```python
from build123d import *

# Parameters (mm, degrees)
SKETCH1_R                 = 3.96875
SKETCH1_R_2               = 1.5875
BODY_DEPTH                = 38.1
SKETCH1_3_R               = 1.5875
POT_SHAFT_OPENING_DEPTH   = 15.24
F_6_32_TAPPED_HOLE1_D     = 2.7051
F_6_32_TAPPED_HOLE1_DEPTH = 3.81
F_6_32_TAPPED_HOLE1_TIP   = 0.81269403


with BuildPart() as part:
    # Sketch1 → Body (new body)
    # profile 1 of 2: a face of its own
    with BuildSketch(Plane.XY):
        Circle(SKETCH1_R)
        Circle(SKETCH1_R_2, mode=Mode.SUBTRACT)
    # profile 2 of 2: a face of its own
    with BuildSketch(Plane.XY):
        Circle(SKETCH1_R_2)
    extrude(amount=-BODY_DEPTH)

    # Sketch1_3 → POT Shaft Opening (cut)
    with BuildSketch(Plane.XY):
        Circle(SKETCH1_3_R)
    extrude(amount=-POT_SHAFT_OPENING_DEPTH, mode=Mode.SUBTRACT)

    # 6-32 Tapped Hole1
    with Locations(Plane(origin=(3.96875, 0, 0), x_dir=(0, 0, -1), z_dir=(1, 0, 0))):
        with Locations((4.7625, 0)):
            Hole(F_6_32_TAPPED_HOLE1_D / 2, depth=F_6_32_TAPPED_HOLE1_DEPTH)
            with Locations((0, 0, -(F_6_32_TAPPED_HOLE1_DEPTH + F_6_32_TAPPED_HOLE1_TIP / 2))):  # 118° drill point
                Cone(0, F_6_32_TAPPED_HOLE1_D / 2, F_6_32_TAPPED_HOLE1_TIP, mode=Mode.SUBTRACT)


solid = part.part
```
Input: part model. Units: mm. Frame: model coordinates. A direction names the side the tool comes from. Round coordinates to 2 decimals unless told otherwise and drop trailing zeros. Order: outer loops, then holes, each group sorted by start corner. A loop starts at its lowest first (then second) coordinate and runs counter-clockwise, first axis right, second up. Notation, with made-up numbers: (-25.75, 16.25) - (19.25, 16.25) arc R15 ccw to (19.25, 32.25) - close; hole circle Ø9 at (42, 6). An arc over 180 degrees is marked (long way). One line per question, with ' | ' between items. Start each with the question number.
1) Contact query for flat-ended pins moving along their axis: P1, Ø1.5, axis at x = 2, z = -13, coming from the +Y side; P2, Ø2, axis at x = -2.5, z = -21, coming from the +Y side. Output: stop coordinate, or through.
2) Set-up query: faces 1 (the flat face through (0, 0, -15.24)), 2 (the flat face through (2, 0, 0)). Return all of +Z, -Z, +X, -X, +Y, -Y with unobstructed straight access to the full face (end or side cutting, diameter ignored); none if empty.
3) Cut plane D-D, the plane x = 2.5. Return the cut outline in (y, z).
4) Pull-direction query (X, two-part tool) for faces 3 (the cylindrical face through (-0.86, -3.874, -18.783)), 4 (the cylindrical face through (-1.586, 0.07, -7.513)), 5 (the cylindrical face through (2.38, 1.34, -4.94)); classes: +X half, -X half, draft (parallel to the pull), parting line (faces both ways), or undercut.
5) Cut plane A-A, the plane y = 0. Return the cut outline in (x, z), then the cut area to 3 significant figures.
6) Cut plane C-C, the plane z = -6.5. Return the cut outline in (x, y) (1 decimal).
7) Cut plane B-B, the plane x = 0. Return the cut outline in (y, z).
8) Ray query, probe 1 along Z at (x, y) = (2.75, 0); probe 2 along Y at (x, z) = (0, -5.75); probe 3 along X at (y, z) = (-0.75, -10). Return the intervals inside material, ascending.
Worked out:
1) P1: stops at y = 3.77 | P2: stops at y = 3.67
2) face 1: +Z | face 2: +Z, +X, -X, +Y, -Y
3) outline: (-3.08, -38.1) - (3.08, -38.1) - (3.08, 0) - (-3.08, 0) - close; hole circle Ø2.71 at (0, -4.76)
4) face 3: parting line | face 4: undercut | face 5: draft
5) outline: (-3.97, -38.1) - (3.97, -38.1) - (3.97, -6.12) - (1.59, -6.12) - (1.59, -15.24) - (-1.59, -15.24) - (-1.59, 0) - (-3.97, 0) - close; (1.59, -3.41) - (3.97, -3.41) - (3.97, 0) - (1.59, 0) - close | area: 248 mm^2
6) outline: circle Ø7.9 at (0, 0); hole circle Ø3.2 at (0, 0)
7) outline: (-3.97, -38.1) - (3.97, -38.1) - (3.97, 0) - (1.59, 0) - (1.59, -15.24) - (-1.59, -15.24) - (-1.59, 0) - (-3.97, 0) - close
8) probe 1: z = -38.1 to -6.12, -3.41 to 0 | probe 2: y = -3.97 to -1.59, 1.59 to 3.97 | probe 3: x = -3.9 to -1.4, 1.4 to 3.9
